Geometry check sheet. Reference: the model listing, model coordinates, mm. Face numbers are marked on the shaded views. A direction names the side the tool comes from. Give positions to 0.01 mm unless a question says otherwise; leave off trailing zeros. Loops run counter-clockwise (first coordinate to the right, second up) from the corner with the lowest first, then second, coordinate; pieces in that order, holes last. Notation, with made-up numbers: (41, 71) -> (78, 71) arc R11 ccw to (78, 88) -> close; hole circle Ø6 at (58, 14). An arc over 180 degrees is marked (long way). Answer as a JSON object with one key per item and string values.
from build123d import *

# Parameters (mm, degrees)
ESBO_O1_R                = 55
RESSALTO_EXTRUS_O1_DEPTH = 25
ESBO_O2_R                = 50
RESSALTO_EXTRUS_O2_DEPTH = 10
CASCA1_T                 = -5
FILETE2_R                = 2
FILETE3_R                = 2
ESBO_O3_R                = 25
ESBO_O3_R_2              = 12.5
CORTE_EXTRUS_O1_DEPTH    = 86.293610546


with BuildPart() as part:
    # Esboço1 → Ressalto-extrusão1 (new body)
    with BuildSketch(Plane.XY):
        Circle(ESBO_O1_R)
    extrude(amount=RESSALTO_EXTRUS_O1_DEPTH)

    # Esboço2 → Ressalto-extrusão2 (add)
    with BuildSketch(Plane(origin=(0, 0, 0), x_dir=(-1, 0, 0), z_dir=(0, 0, -1))):
        Circle(ESBO_O2_R)
    extrude(amount=RESSALTO_EXTRUS_O2_DEPTH)

    # Casca1
    casca1_openings = [part.faces().sort_by_distance(p)[0] for p in [
        (0, 0, 25),
    ]]
    offset(amount=CASCA1_T, openings=casca1_openings, kind=Kind.INTERSECTION)

    # Filete2
    filete2_edges = [part.edges().sort_by_distance(p)[0] for p in [
        (50, 0, 0),
        (50, 0, -10),
    ]]
    fillet(filete2_edges, radius=FILETE2_R)

    # Filete3
    filete3_edges = [part.edges().sort_by_distance(p)[0] for p in [
        (-55, 0, 0),
    ]]
    fillet(filete3_edges, radius=FILETE3_R)

    # Esboço3 → Corte-extrusão1 (cut, through all)
    with BuildSketch(Plane(origin=(0, 0, -10), x_dir=(-1, 0, 0), z_dir=(0, 0, -1))):
        with Locations((0, 18)):
            Circle(ESBO_O3_R)
        with Locations((0, -28)):
            Circle(ESBO_O3_R_2)
    extrude(amount=-CORTE_EXTRUS_O1_DEPTH, mode=Mode.SUBTRACT)


solid = part.part
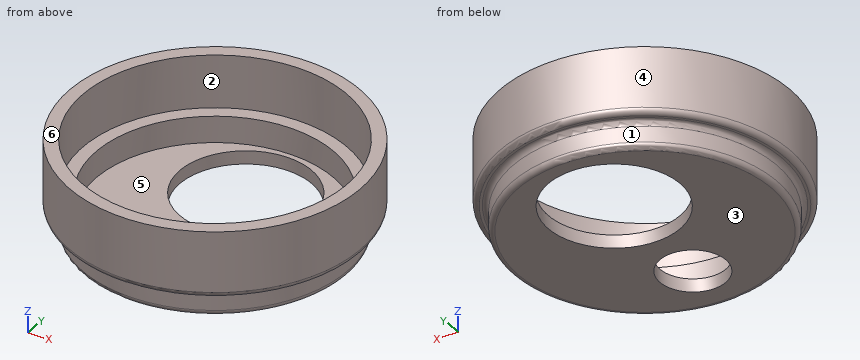
1) Section check B-B on y = 0. Record the cut outline in (x, z).
Geometry check:
{"outline": "(-55, 2) arc R2 ccw to (-53, 0) -> (-52, 0) arc R2 cw to (-50, -2) -> (-50, -8) arc R2 ccw to (-48, -10) -> (-17.35, -10) -> (-17.35, -5) -> (-45, -5) -> (-45, 5) -> (-50, 5) -> (-50, 25) -> (-55, 25) -> close; (17.35, -10) -> (48, -10) arc R2 ccw to (50, -8) -> (50, -2) arc R2 cw to (52, 0) -> (53, 0) arc R2 ccw to (55, 2) -> (55, 25) -> (50, 25) -> (50, 5) -> (45, 5) -> (45, -5) -> (17.35, -5) -> close"}
2) Material ranges on line 1 along Y through (x, z) = (0, 20.25); line 2 along Y through (x, z) = (0, -3); line 3 along Z through (x, y) = (-35, 31), recorded low to high. Write a range as from..to.
Geometry check:
{"line 1": "y = -55..-50, 50..55", "line 2": "y = -50..-45, 45..50", "line 3": "z = -10..5"}
3) Draft check along Y on the marked faces 4, 5 and 6. Enter one of: pulls with the +Y half, pulls with the -Y half, needs draft (parallel to the pull), parting line crosses it, or undercut.
Geometry check:
{"face 4": "parting line crosses it", "face 5": "undercut", "face 6": "needs draft"}
4) Section check A-A on x = 0. Count the separate pieces of the cut face and the enclosed holes in it, plus the area to 3 significant figures.
Geometry check:
{"separate pieces": "3", "enclosed holes": "0", "area": "473 mm2"}
5) Tool access check on the marked faces 1, 2 and 3. Record the directions out of +Z, -Z, +X, -X, +Y, -Y that give a thin tool (end or side, any length) a straight path to the whole face; none if there is none.
Geometry check:
{"face 1": "-Z", "face 2": "+Z", "face 3": "-Z, +X, -X, +Y, -Y"}
6) Depth check by flat-ended pin: P1, Ø1.5, axis at x = -14, y = -33, coming from the +Z side; P2, Ø1, axis at y = -39, z = 20, coming from the +X side; P3, Ø10, axis at x = 10.5, z = 4, coming from the +Y side. Enter the tip coordinate at first touch or a pass-through.
Geometry check:
{"P1": "stops at z = -5", "P2": "stops at x = 39.28", "P3": "stops at y = 54.72"}
7) Section check C-C on z = 21. Record the cut outline in (x, y), plus the area to 3 significant figures.
Geometry check:
{"outline": "circle Ø110 at (0, 0); hole circle Ø100 at (0, 0)", "area": "1,650 mm2"}
